from build123d import *

# Parameters (mm, degrees)
SKETCH3_R           = 38.1
SKETCH3_R_2         = 28.575
BOSS_EXTRUDE1_DEPTH = 69.85
SKETCH4_W           = 19.05
SKETCH4_H           = 2.54
CHAMFER1_SIZE       = 8.89


with BuildPart() as part:
    # Sketch3 → Boss-Extrude1 (new, symmetric)
    with BuildSketch(Plane.XY):
        Circle(SKETCH3_R)
        Circle(SKETCH3_R_2, mode=Mode.SUBTRACT)
    extrude(amount=BOSS_EXTRUDE1_DEPTH, both=True)

    # Sketch4 → Cut-Revolve1 (revolve, cut)
    with BuildSketch(Plane(origin=(0, 0, 0), x_dir=(0, 0, -1), z_dir=(1, 0, 0)), mode=Mode.PRIVATE) as cut_revolve1_sk:
        with Locations((-33.853856194, 36.83)):
            Rectangle(SKETCH4_W, SKETCH4_H)
        with Locations((33.853856194, 36.83)):
            Rectangle(SKETCH4_W, SKETCH4_H)
    revolve(cut_revolve1_sk.sketch.rotate(Axis((0, 0, 69.85), (0, 0, -1)), 180), axis=Axis((0, 0, 69.85), (0, 0, -1)), mode=Mode.SUBTRACT)

    # Chamfer1
    chamfer1_edges = [part.edges().sort_by_distance(p)[0] for p in [
        (-28.575, 0, 69.85),
    ]]
    chamfer(chamfer1_edges, length=CHAMFER1_SIZE)


solid = part.part
Input: part model. Units: mm. Frame: model coordinates. A direction names the side the tool comes from. Coordinates: 2 decimals unless noted, no trailing zeros. Loops run counter-clockwise (first coordinate to the right, second up) from the corner with the lowest first, then second, coordinate; pieces in that order, holes last. Notation, with made-up numbers: (-15.5, 49) -> (18.5, 49) arc R17 ccw to (18.5, 59) -> close; hole circle Ø2 at (61.5, 77.25). An arc over 180 degrees is marked (long way). Write item = value, one per line. Start each with the question number.
Item 1: First-contact query: P1, Ø5, axis at y = -6, z = -13.5, coming from the +X side; P2, Ø1.5, axis at y = -5.5, z = 17.5, coming from the -X side; P3, Ø23, axis at x = -17, y = -4, coming from the +Z side; P4, Ø12, axis at y = -6, z = -2, coming from the +X side. Flat tips, straight axial feed; report the tip coordinate or a pass-through.
Item 2: Reachability of faces 4 (the face through (5.5, 28.4, -69.85)), 5 (the face through (34.714, 7.709, 33.721)) from +Z, -Z, +X, -X, +Y, -Y: full face, straight path, thin tool, end or side. Return the list, or none.
Item 3: Cut plane A-A, the plane x = 0. Return loops of the section in (y, z) (3 decimals).
Item 4: Mould query, pull axis X, two halves, no side actions, for faces 1 (the face through (34.714, 7.709, -33.987)), 2 (the face through (-28.547, 1.256, -5.361)), 3 (the face through (34, -11, 24.329)). Classes: pulls with the +X half, pulls with the -X half, needs draft (parallel to the pull), parting line crosses it, or undercut.
Item 5: Cut plane D-D, the plane z = -18. Return loops of the section in (x, y) (3 decimals), plus the area to 3 significant figures.
Item 6: Material intervals for line 1 (Y direction, x = 0, z = 2.5) (3 decimals); line 2 (Z direction, x = -22, y = -28.5); line 3 (X direction, y = -3, z = 39.5), sorted ascending.
Item 7: Cut plane C-C, the plane z = 40.5. Return loops of the section in (x, y) (3 decimals).
Ans:
q1.P1 = 37.94
q1.P2 = -37.8
q1.P3 = 61.35
q1.P4 = 38.1
q2.face_4 = -Z, +X, -X, +Y, -Y
q2.face_5 = none
q3.outline = (-38.1, -69.85) -> (-28.575, -69.85) -> (-28.575, 60.96) -> (-37.465, 69.85) -> (-38.1, 69.85) -> (-38.1, 43.379) -> (-35.56, 43.379) -> (-35.56, 24.329) -> (-38.1, 24.329) -> (-38.1, -24.329) -> (-35.56, -24.329) -> (-35.56, -43.379) -> (-38.1, -43.379) -> close; (28.575, -69.85) -> (38.1, -69.85) -> (38.1, -43.379) -> (35.56, -43.379) -> (35.56, -24.329) -> (38.1, -24.329) -> (38.1, 24.329) -> (35.56, 24.329) -> (35.56, 43.379) -> (38.1, 43.379) -> (38.1, 69.85) -> (37.465, 69.85) -> (28.575, 60.96) -> close
q4.face_1 = parting line crosses it
q4.face_2 = undercut
q4.face_3 = needs draft
q5.outline = circle Ø76.2 at (0, 0); hole circle Ø57.15 at (0, 0)
q5.area = 2,000 mm²
q6.line_1 = -38.1 to -28.575, 28.575 to 38.1
q6.line_2 = -69.85 to -43.38, -24.33 to 24.33, 43.38 to 68.39
q6.line_3 = -35.43 to -28.42, 28.42 to 35.43
q7.outline = circle Ø71.12 at (0, 0); hole circle Ø57.15 at (0, 0)
